```python
from build123d import *

# Parameters (mm, degrees)
F0_W      = 60
F0_H      = 40
F1_DEPTH  = 5
F2_W      = 5
F2_H      = 30
F3_DEPTH  = 10
F5_DEPTH  = 25
F6_R      = 3.9
F7_DEPTH  = 5.2
F8_R      = 7
F9_DEPTH  = 3
F9_TAPER  = 25
F10_W     = 1.5
F10_H     = 1.5
F10_W_2   = 7.1590355843
F10_H_2   = 7.6815277636
F11_DEPTH = 7
F12_DEPTH = 7
F14_DEPTH = 8
F15_R     = 3
F16_DEPTH = 25


with BuildPart() as f1:
    # F0 (on Top) → F1 (new body)
    with BuildSketch(Plane.XY):
        Rectangle(F0_W, F0_H)
    extrude(amount=F1_DEPTH)

    # F2 (on face) → F3 (join)
    with BuildSketch(Plane.XY.offset(5)):
        Polygon((30, 20), (-30, 20), (-30, 15), (-25, 15), (25, 15), (30, 15), align=None)
        with Locations((-27.5, 0)):
            Rectangle(F2_W, F2_H)
        Polygon((30, -20), (30, 15), (25, 15), (25, -15), (25, -20), align=None)
        Polygon((-25, -15), (-30, -15), (-30, -20), (25, -20), (25, -15), align=None)
    extrude(amount=F3_DEPTH)

    # F4 (on face) → F5 (cut)
    with BuildSketch(Plane(origin=(0, 0, 0), x_dir=(1, 0, 0), z_dir=(0, 0, -1))):
        with BuildLine():
            Line((25, 0), (30, 0))
            Line((30, 0), (30, 20))
            Line((30, 20), (10, 20))
            Line((10, 20), (10, 15))
            ThreePointArc((10, 15), (14.3933982822, 4.3933982822), (25, 0))
        make_face()
    extrude(amount=-F5_DEPTH, mode=Mode.SUBTRACT)

    # F6 (on face) → F7 (join)
    with BuildSketch(Plane.XY.offset(5)):
        with Locations((11.9, 0)):
            Circle(F6_R)
        with Locations((-11.9, 0)):
            Circle(F6_R)
    extrude(amount=F7_DEPTH)

    # F8 (on face) → F9 (join)
    with BuildSketch(Plane.XY.offset(10.2)):
        with Locations((-11.9, 0)):
            Circle(F8_R)
        with Locations((11.9, 0)):
            Circle(F8_R)
    extrude(amount=F9_DEPTH, taper=F9_TAPER)

    # F10 (on face) → F11 (cut)
    with BuildSketch(Plane.XY.offset(13.2)):
        Polygon((-11.15, 7.5554959476), (-11.9, 7.5554959476), (-12.65, 7.5554959476), (-12.65, 0.75), (-11.15, 0.75), align=None)
        Polygon((-2.854565857, 0.75), (-11.15, 0.75), (-11.15, -0.75), (-2.854565857, -0.75), (-2.854565857, 0), align=None)
        with Locations((-11.9, 0)):
            Rectangle(F10_W, F10_H)
        with Locations((-16.2295177922, 0)):
            Rectangle(F10_W_2, F10_H)
        with Locations((-11.9, -4.5907638818)):
            Rectangle(F10_W, F10_H_2)
        Polygon((12.65, 0.75), (12.65, 7.5554959476), (11.9, 7.5554959476), (11.15, 7.5554959476), (11.15, 0.75), align=None)
        with Locations((16.2295177922, 0)):
            Rectangle(F10_W_2, F10_H)
        with Locations((11.9, 0)):
            Rectangle(F10_W, F10_H)
        with Locations((11.9, -4.5907638818)):
            Rectangle(F10_W, F10_H_2)
        Polygon((11.15, -0.75), (11.15, 0.75), (2.854565857, 0.75), (2.854565857, 0), (2.854565857, -0.75), align=None)
    extrude(amount=-F11_DEPTH, mode=Mode.SUBTRACT)

    # F10 (on face) → F12 (cut)
    with BuildSketch(Plane.XY.offset(13.2)):
        Polygon((-11.15, 7.5554959476), (-11.9, 7.5554959476), (-12.65, 7.5554959476), (-12.65, 0.75), (-11.15, 0.75), align=None)
        Polygon((-2.854565857, 0.75), (-11.15, 0.75), (-11.15, -0.75), (-2.854565857, -0.75), (-2.854565857, 0), align=None)
        with Locations((-11.9, 0)):
            Rectangle(F10_W, F10_H)
        with Locations((-16.2295177922, 0)):
            Rectangle(F10_W_2, F10_H)
        with Locations((-11.9, -4.5907638818)):
            Rectangle(F10_W, F10_H_2)
        Polygon((12.65, 0.75), (12.65, 7.5554959476), (11.9, 7.5554959476), (11.15, 7.5554959476), (11.15, 0.75), align=None)
        with Locations((16.2295177922, 0)):
            Rectangle(F10_W_2, F10_H)
        with Locations((11.9, 0)):
            Rectangle(F10_W, F10_H)
        with Locations((11.9, -4.5907638818)):
            Rectangle(F10_W, F10_H_2)
        Polygon((11.15, -0.75), (11.15, 0.75), (2.854565857, 0.75), (2.854565857, 0), (2.854565857, -0.75), align=None)
    extrude(amount=-F12_DEPTH, mode=Mode.SUBTRACT)

    # F13 (on face) → F14 (join)
    with BuildSketch(Plane(origin=(0, 0, 0), x_dir=(1, 0, 0), z_dir=(0, 0, -1))):
        Polygon((-23.4916425814, -19.4916425814), (-29.4916425814, -13.4916425814), (-37.225079692, -21.225079692), (-31.225079692, -27.225079692), align=None)
        Polygon((-31.225079692, -27.225079692), (-37.225079692, -21.225079692), (-40.7606135979, -24.7606135979), (-34.7606135979, -30.7606135979), align=None)
    extrude(amount=-F14_DEPTH)

    # F15 (on face) → F16 (cut)
    with BuildSketch(Plane.XY.offset(8)):
        with Locations((-34.1515289412, 24.1206135979)):
            Circle(F15_R)
    extrude(amount=-F16_DEPTH, mode=Mode.SUBTRACT)


solid = f1.part
```
The listing builds one solid part. Answer for the finished solid, in the listing's coordinates (mm). A direction names the side the tool comes from. Coordinates: 2 decimals unless noted, no trailing zeros. Write each loop counter-clockwise with the first axis right and the second up, starting at its lowest first coordinate (ties: lowest second). Pieces come first, ordered by that corner, then holes. Notation, with made-up numbers: (3, 16.5) - (25, 16.5) arc R23 cw to (25, 42.5) - close; hole circle Ø1 at (62, 66.25). An arc over 180 degrees is marked (long way). One line per item, written item: value.
1) Consider line 1 along X through (y, z) = (3, 9.75); line 2 along X through (y, z) = (-3, 6); line 3 along Y through (x, z) = (26.5, 9.25). Determine where each line is inside the solid, lowest interval first. Write a range as from..to.
Geometry check:
line 1: x = -30..-25, -14.39..-12.65, -11.15..-9.41, 9.41..11.15, 12.65..14.39, 25..30
line 2: x = -30..-25, -14.39..-9.41, 9.41..14.39
line 3: y = 0..20
2) Find section A-A (z = 14). Give the vertices of the cut face in (x, y).
Geometry check:
outline: (-30, -20) - (10, -20) - (10, -15) - (-25, -15) - (-25, 15) - (25, 15) - (25, 0) - (30, 0) - (30, 20) - (-30, 20) - close
3) Find section D-D (y = 9). Give the vertices of the cut face in (x, z).
Geometry check:
outline: (-30, 0) - (30, 0) - (30, 15) - (25, 15) - (25, 5) - (-25, 5) - (-25, 15) - (-30, 15) - close
4) Find section B-B (x = -11.9). Give the vertices of the cut face in (y, z), and give its area (3 significant figures).
Geometry check:
outline: (-20, 0) - (20, 0) - (20, 15) - (15, 15) - (15, 5) - (3.9, 5) - (3.9, 6.2) - (-3.9, 6.2) - (-3.9, 5) - (-15, 5) - (-15, 15) - (-20, 15) - close
area: 309 mm2
5) A tool of negligible diameter and unlimited length cuts with its end or side. For faces 1 (the flat face through (14, 3, 13.2)), 2 (the conical face through (16.28, 4.3, 12.05)), 3 (the flat face through (-8, 4, 10.2)), from which of +Z, -Z, +X, -X, +Y, -Y can it reach the whole face along a straight path? Write none if from no direction.
Geometry check:
face 1: +Z, -Y
face 2: +Z
face 3: none
6) Each of these flat-tipped pins is pushed along its axis until it touches: pin 1 Ø7 at (x, z) = (15, 9.5) entering from -Y; pin 2 Ø5 at (x, z) = (-9.5, 4) entering from +Y; pin 3 Ø1.5 at (x, z) = (28, 11) entering from -Y; pin 4 Ø6 at (x, y) = (21, -5.5) entering from -Z (3 decimals). Where does it stop, or does it pass through?
Geometry check:
pin 1: stops at y = -6.96
pin 2: stops at y = 20
pin 3: stops at y = 0
pin 4: passes through
7) Find section C-C (z = 2.25). Give the vertices of the cut face in (x, y), and give its area (3 significant figures).
Geometry check:
outline: (-40.76, 24.76) - (-30, 14) - (-30, -20) - (10, -20) - (10, -15) arc R15 cw to (25, 0) - (30, 0) - (30, 20) - (-24, 20) - (-34.76, 30.76) - close; hole circle Ø6 at (-34.15, 24.12)
area: 2,130 mm2
